Autodesk Inventor part; units mm, degrees
ref_plane "YZ Plane" through (0, 0, 0) normal (1, 0, 0) x (0, 1, 0)
ref_plane "XZ Plane" through (0, 0, 0) normal (0, 1, 0) x (-1, 0, 0)
ref_plane "XY Plane" through (0, 0, 0) normal (0, 0, 1) x (1, 0, 0)
sketch "Sketch1" plane through (0, 0, 0) normal (0, 1, 0) x (-1, 0, 0)
  line L0 (-350, 675) -> (350, 675)
  line L1 (350, 675) -> (350, -675)
  line L2 (350, -675) -> (-350, -675)
  line L3 (-350, -675) -> (-350, 675)
  line L4 (-350, 675) -> (350, -675) construction
  line L5 (350, 675) -> (-350, -675) construction
  line L6 (350, 675) -> (-350, 675)
  line L7 (-350, 675) -> (-350, 325)
  line L8 (-350, 325) -> (350, 325)
  line L9 (350, 325) -> (350, 675)
  line L10 (350, 325) -> (-350, 325)
  line L11 (-350, 325) -> (-350, -75)
  line L12 (-350, -75) -> (350, -75)
  line L13 (350, -75) -> (350, 325)
  line L14 (350, -75) -> (-350, -75)
  line L15 (-350, -75) -> (-350, -425)
  line L16 (-350, -425) -> (350, -425)
  line L17 (350, -425) -> (350, -75)
  line L18 (350, -425) -> (-350, -425)
  line L19 (-350, -425) -> (-350, -675)
  line L20 (-350, -675) -> (350, -675)
  line L21 (350, -675) -> (350, -425)
  point P0 (0, 0)
  dimension "d1" = 1350
  dimension "d2" = 700
  dimension "d3" = 350
  dimension "d4" = 400
  dimension "d5" = 350
extrude "Extrusion1" add sketch "Sketch1" along normal blind 50 contours L0 L1 L8 L3
extrude "Extrusion2" add sketch "Sketch1" along normal blind 30 contours L8 L1 L12 L3
extrude "Extrusion3" add sketch "Sketch1" along normal blind 90 contours L12 L1 L16 L3
extrude "Extrusion4" add sketch "Sketch1" along normal blind 70 contours L16 L1 L2 L3
sketch "Sketch2" plane through (0, 90, 0) normal (0, 1, 0) x (1, 0, 0)
  line L0 (-320, 105) -> (320, 105)
  line L1 (320, 105) -> (320, 395)
  line L2 (320, 395) -> (-320, 395)
  line L3 (-320, 395) -> (-320, 105)
  line L4 (-350, 75) -> (350, 75)
  line L5 (-350, 425) -> (-350, 75)
  line L6 (350, 75) -> (350, 425)
  line L7 (350, 425) -> (-350, 425)
  line L8 (-245, 485) -> (-115, 485)
  line L9 (-115, 485) -> (-115, 615)
  line L10 (-115, 615) -> (-245, 615)
  line L11 (-245, 615) -> (-245, 485)
  line L12 (-65, 485) -> (65, 485)
  line L13 (65, 485) -> (65, 615)
  line L14 (65, 615) -> (-65, 615)
  line L15 (-65, 615) -> (-65, 485)
  line L16 (115, 485) -> (245, 485)
  line L17 (245, 485) -> (245, 615)
  line L18 (245, 615) -> (115, 615)
  line L19 (115, 615) -> (115, 485)
  line L20 (-350, 675) -> (-350, 425)
  point P0 (0, 0)
  point P1 (320, 250)
  dimension "d14" = 30
  dimension "d15" = 30
  dimension "d16" = 30
  dimension "d17" = 30
  dimension "d18" = 130
  dimension "d19" = 130
  dimension "d20" = 105
  dimension "d21" = 60
  dimension "d22" = 50
  dimension "d23" = 50
extrude "Extrusion5" cut sketch "Sketch2" against normal blind 70 contours L3 L2 L1 L0
extrude "Extrusion6" cut sketch "Sketch2" against normal blind 50 contours L11 L10 L9 L8 | L15 L14 L13 L12 | L19 L18 L17 L16
sketch "Sketch4" plane through (0, 0, 0) normal (0, -1, 0) x (1, 0, 0)
  line L0 (-350, -675) -> (-350, 675)
  line L1 (-350, 675) -> (-320, 675)
  line L2 (-320, 675) -> (-320, 645)
  line L3 (-320, 645) -> (-350, 645)
  line L4 (-350, 645) -> (-350, 675)
  line L5 (-350, 675) -> (350, 675)
  line L6 (350, 675) -> (350, -675)
  line L7 (320, 675) -> (350, 675)
  line L8 (350, 675) -> (350, 645)
  line L9 (350, 645) -> (320, 645)
  line L10 (320, 645) -> (320, 675)
  line L11 (-350, -675) -> (-350, -425)
  line L12 (-350, -675) -> (-320, -675)
  line L13 (-320, -675) -> (-320, -645)
  line L14 (-320, -645) -> (-350, -645)
  line L15 (-350, -645) -> (-350, -675)
  line L16 (350, -675) -> (320, -675)
  line L17 (320, -675) -> (320, -645)
  line L18 (320, -645) -> (350, -645)
  line L19 (350, -645) -> (350, -675)
  line L20 (-15, 675) -> (15, 675)
  line L21 (15, 675) -> (15, 645)
  line L22 (15, 645) -> (-15, 645)
  line L23 (-15, 645) -> (-15, 675)
  line L24 (350, -675) -> (-350, -675)
  line L25 (-15, -675) -> (15, -675)
  line L26 (15, -675) -> (15, -645)
  line L27 (15, -645) -> (-15, -645)
  line L28 (-15, -645) -> (-15, -675)
  line L29 (-350, 15) -> (-320, 15)
  line L30 (-320, 15) -> (-320, -15)
  line L31 (-320, -15) -> (-350, -15)
  line L32 (-350, -15) -> (-350, 15)
  line L33 (320, 15) -> (350, 15)
  line L34 (350, 15) -> (350, -15)
  line L35 (350, -15) -> (320, -15)
  line L36 (320, -15) -> (320, 15)
  line L37 (-15, 15) -> (15, 15)
  line L38 (15, 15) -> (15, -15)
  line L39 (15, -15) -> (-15, -15)
  line L40 (-15, -15) -> (-15, 15)
  point P0 (0, 0)
  point P1 (0, -645)
  point P2 (0, -675)
  point P3 (0, 645)
  point P4 (320, 0)
  point P5 (-320, 0)
  point P6 (-350, 0)
  point P7 (350, 0)
  point P8 (0, 15)
  point P9 (15, 0)
  dimension "d32" = 30
  dimension "d33" = 30
extrude "Extrusion8" add sketch "Sketch4" along normal blind 500 contours L0 L14 L13 L12 | L28 L27 L26 L24 | L0 L29 L30 L31 | L17 L18 L6 L16 | L0 L1 L2 L3 | L35 L36 L33 L6 | L5 L21 L22 L23 | L9 L10 L5 L6 | L37 L38 L39 L40
sketch "Sketch5" plane through (0, 30, 0) normal (0, 1, 0) x (1, 0, 0)
  line L0 (-350, 75) -> (-350, -325)
  line L1 (350, -325) -> (350, 75)
  line L2 (-350, -25) -> (350, -25)
  line L3 (350, -25) -> (350, -75)
  line L4 (350, -75) -> (-350, -75)
  line L5 (-350, -75) -> (-350, -25)
  line L6 (-350, -175) -> (350, -175)
  line L7 (350, -175) -> (350, -225)
  line L8 (350, -225) -> (-350, -225)
  line L9 (-350, -225) -> (-350, -175)
  line L10 (350, -325) -> (-350, -325)
  line L11 (-350, 75) -> (350, 75)
  point P0 (0, 0)
  point P1 (350, -25)
  point P2 (-350, -225)
  point P3 (350, -175)
  dimension "d36" = 700
  dimension "d37" = 50
  dimension "d38" = 50
  dimension "d39" = 100
  dimension "d40" = 100
extrude "Extrusion9" add sketch "Sketch5" along normal blind 50 contours L2 L1 L4 L0 | L6 L1 L8 L0
properties part number "Table"
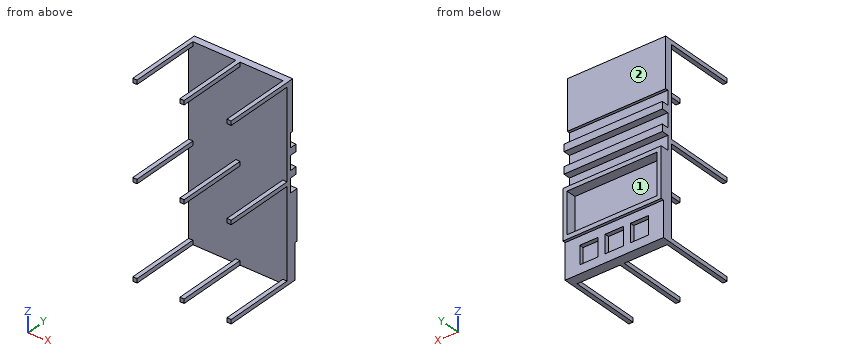
For this review, take the finished solid that the model builds, in its own axes (mm). Face numbers are marked on the shaded views. Coordinates: 2 decimals unless noted, no trailing zeros. Write each loop counter-clockwise with the first axis right and the second up, starting at its lowest first coordinate (ties: lowest second). Pieces come first, ordered by that corner, then holes. Notation, with made-up numbers: (40.25, -12.5) - (94.25, -12.5) arc R23 cw to (94.25, 5.5) - close; hole circle Ø2 at (53, 44.25). An arc over 180 degrees is marked (long way). Put each result on its own line as item: value.
1. Add section C-C, the plane y = -207. Count the separate pieces of the cut face and the enclosed holes in it, then the cut area to 3 significant figures.
Values found:
separate pieces: 9
enclosed holes: 0
area: 8,100 mm²
2. Add section D-D, the plane z = 354.5. Give the boundary of the cut face in (x, y).
Values found:
outline: (-350, 0) - (350, 0) - (350, 50) - (-350, 50) - close
3. For pin 1 (4 mm diameter, centred on x = 181, z = 485.5, fed in from -Y); pin 2 (4 mm diameter, centred on x = -114.5, z = 403, fed in from +Y); pin 3 (5 mm diameter, centred on x = 155.5, z = 294.5, fed in from +Y), all flat-tipped, find the tip position at first contact; note any pin that passes through.
Values found:
pin 1: y = 0
pin 2: y = 50
pin 3: y = 30
4. Add section B-B, the plane x = -51.5. Give the boundary of the cut face in (y, z), then the cut area to 3 significant figures.
Values found:
outline: (0, -675) - (70, -675) - (70, -615) - (40, -615) - (40, -485) - (70, -485) - (70, -425) - (90, -425) - (90, -395) - (20, -395) - (20, -105) - (90, -105) - (90, -75) - (30, -75) - (30, 25) - (80, 25) - (80, 75) - (30, 75) - (30, 175) - (80, 175) - (80, 225) - (30, 225) - (30, 325) - (50, 325) - (50, 675) - (0, 675) - close
area: 59,300 mm²
5. Wall thickness on probe 1 along Z at (x, y) = (305.5, 46.5); probe 2 along Z at (x, y) = (-117, 62); probe 3 along X at (y, z) = (-406, -2): over which ranges is each line inside the solid? List them lowest first.
Values found:
probe 1: -675 to -395, -105 to -75, 25 to 75, 175 to 225, 325 to 675
probe 2: -675 to -615, -485 to -395, -105 to -75, 25 to 75, 175 to 225
probe 3: -350 to -320, -15 to 15, 320 to 350
6. Mouldability with a two-part tool opening along X and no side actions: class the marked faces 1 and 2 as released by +X, released by -X, zero draft, split by the parting line, or undercut.
Values found:
face 1: undercut
face 2: zero draft
7. Add section A-A, the plane z = -223.5. Give the boundary of the cut face in (x, y), then the cut area to 3 significant figures.
Values found:
outline: (-350, 0) - (350, 0) - (350, 90) - (320, 90) - (320, 20) - (-320, 20) - (-320, 90) - (-350, 90) - close
area: 18,200 mm²
